```python
from build123d import *

# Parameters (mm, degrees)
SKETCH1_R      = 1
EXTRUDE2_DEPTH = 5
FILLET2_R      = 3.5
FILLET3_R      = 1.5
EXTRUDE4_DEPTH = 5
FILLET4_R      = 0.2
EXTRUDE5_DEPTH = 5
FILLET5_R      = 0.2


with BuildPart() as part:
    # Sketch1 → Extrude2 (new body)
    with BuildSketch(Plane.XY):
        with BuildLine():
            Line((-30.522603834, 36.180351438), (-30.522603834, 45.180351438))
            Line((-30.522603834, 45.180351438), (-25.522603834, 45.180351438))
            Line((-25.522603834, 45.180351438), (-7.022603834, 0.180351438))
            Line((-7.022603834, 0.180351438), (-30.522603834, 0.180351438))
            Line((-30.522603834, 0.180351438), (-30.522603834, 10.180351438))
            ThreePointArc((-30.522603834, 10.180351438), (-27.540232283, 23.180351438), (-30.522603834, 36.180351438))
        make_face()
        with Locations((-23.522603834, 3.680351438)):
            Circle(SKETCH1_R, mode=Mode.SUBTRACT)
        with Locations((-11.522603834, 3.680351438)):
            Circle(SKETCH1_R, mode=Mode.SUBTRACT)
    extrude(amount=EXTRUDE2_DEPTH)

    # Fillet2
    fillet2_edges = [part.edges().sort_by_distance(p)[0] for p in [
        (-7.022603834, 0.180351438, 2.5),
    ]]
    fillet(fillet2_edges, radius=FILLET2_R)

    # Fillet3
    fillet3_edges = [part.edges().sort_by_distance(p)[0] for p in [
        (-25.522603834, 45.180351438, 2.5),
    ]]
    fillet(fillet3_edges, radius=FILLET3_R)

    # Sketch3 → Extrude4 (cut)
    with BuildSketch(Plane.XY.offset(5)):
        Polygon((-29.822603834, 43.080351438), (-30.522603834, 43.780351438), (-30.522603834, 42.380351438), align=None)
        Polygon((-29.822603834, 44.480351438), (-30.522603834, 45.180351438), (-30.522603834, 43.780351438), align=None)
        Polygon((-29.822603834, 41.680351438), (-30.522603834, 42.380351438), (-30.522603834, 40.980351438), align=None)
        Polygon((-29.822603834, 40.280351438), (-30.522603834, 40.980351438), (-30.522603834, 39.580351438), align=None)
        Polygon((-29.822603834, 38.880351438), (-30.522603834, 39.580351438), (-30.522603834, 38.180351438), align=None)
        Polygon((-29.822603834, 37.480351438), (-30.522603834, 38.180351438), (-30.522603834, 36.780351438), align=None)
    extrude(amount=-EXTRUDE4_DEPTH, mode=Mode.SUBTRACT)

    # Fillet4
    fillet4_edges = [part.edges().sort_by_distance(p)[0] for p in [
        (-30.522603834, 45.180351438, 2.5),
        (-29.822603834, 43.080351438, 2.5),
        (-30.522603834, 42.380351438, 2.5),
        (-30.522603834, 43.780351438, 2.5),
        (-29.822603834, 44.480351438, 2.5),
        (-29.822603834, 41.680351438, 2.5),
        (-30.522603834, 40.980351438, 2.5),
        (-29.822603834, 40.280351438, 2.5),
        (-30.522603834, 39.580351438, 2.5),
        (-29.822603834, 38.880351438, 2.5),
        (-30.522603834, 38.180351438, 2.5),
        (-29.822603834, 37.480351438, 2.5),
        (-30.522603834, 36.780351438, 2.5),
    ]]
    fillet(fillet4_edges, radius=FILLET4_R)

    # Sketch4 → Extrude5 (cut)
    with BuildSketch(Plane.XY.offset(5)):
        Polygon((-29.822603834, 1.080351438), (-30.522603834, 1.780351438), (-30.522603834, 0.380351438), align=None)
        Polygon((-29.822603834, 2.480351438), (-30.522603834, 3.180351438), (-30.522603834, 1.780351438), align=None)
        Polygon((-29.822603834, 3.880351438), (-30.522603834, 4.580351438), (-30.522603834, 3.180351438), align=None)
        Polygon((-29.822603834, 5.280351438), (-30.522603834, 5.980351438), (-30.522603834, 4.580351438), align=None)
        Polygon((-29.822603834, 6.680351438), (-30.522603834, 7.380351438), (-30.522603834, 5.980351438), align=None)
        Polygon((-29.822603834, 8.080351438), (-30.522603834, 8.780351438), (-30.522603834, 7.380351438), align=None)
        Polygon((-29.822603834, 9.480351438), (-30.522603834, 10.180351438), (-30.522603834, 8.780351438), align=None)
    extrude(amount=-EXTRUDE5_DEPTH, mode=Mode.SUBTRACT)

    # Fillet5
    fillet5_edges = [part.edges().sort_by_distance(p)[0] for p in [
        (-30.522603834, 10.180351438, 2.5),
        (-29.822603834, 2.480351438, 2.5),
        (-30.522603834, 1.780351438, 2.5),
        (-29.822603834, 3.880351438, 2.5),
        (-30.522603834, 3.180351438, 2.5),
        (-29.822603834, 5.280351438, 2.5),
        (-30.522603834, 4.580351438, 2.5),
        (-29.822603834, 6.680351438, 2.5),
        (-30.522603834, 5.980351438, 2.5),
        (-29.822603834, 8.080351438, 2.5),
        (-30.522603834, 7.380351438, 2.5),
        (-29.822603834, 9.480351438, 2.5),
        (-30.522603834, 8.780351438, 2.5),
        (-29.822603834, 1.080351438, 2.5),
        (-30.522603834, 0.380351438, 2.5),
    ]]
    fillet(fillet5_edges, radius=FILLET5_R)


solid = part.part
```
Design review of the part built by this model. Coordinates are the model's own, in mm. Coordinates: 2 decimals unless noted, no trailing zeros. Order: outer loops, then holes, each group sorted by start corner. A loop starts at its lowest first (then second) coordinate and runs counter-clockwise, first axis right, second up. Notation, with made-up numbers: (34, -38) -> (55, -38) arc R13 ccw to (55, -16) -> close; hole circle Ø8 at (47, 1.25). An arc over 180 degrees is marked (long way). One line per item, written item: value. Start each with the question number.
Q1. Take a section at D-D, the plane z = 1.15. Give the number of separate pieces and of enclosed holes in the cut face, then the cut area to 3 significant figures.
Q2. Insertion check: pin 1 Ø1 at (x, z) = (-21, 4.5) entering from +Y; pin 2 Ø1 at (y, z) = (10.5, 1) entering from +X. Each pin has a flat end and moves straight along its axis. Give the tip position at first contact, or say it passes through.
Q3. For probe 1 along X at (y, z) = (4.5, 2.8); probe 2 along X at (y, z) = (3.5, 0.8); probe 3 along Y at (x, z) = (-24.25, 4.65), list the stretches that pass through material, from the lowest coordinate up.
Q4. Take a section at C-C, the plane y = 23. State the section outline as (x, z) points, then the cut area to 3 significant figures.
Q5. Take a section at A-A, the plane x = -11.5. State the section outline as (y, z) points, then the cut area to 3 significant figures.
Q6. Mouldability with a two-part tool opening along X and no side actions: class faces 1 (the flat face through (-22, 18, 5)), 2 (the cylindrical face through (-25.68, 44.92, 2.54)), 3 (the cylindrical face through (-27.54, 23.06, 2.46)), 4 (the cylindrical face through (-10.599, 3.297, 2.465)) as pulls with the +X half, pulls with the -X half, needs draft (parallel to the pull), parting line crosses it, or undercut.
Q7. Take a section at B-B, the plane x = -28.25. State the section outline as (y, z) points.
Values follow:
1. separate pieces: 1
1. enclosed holes: 2
1. area: 570 mm2
2. pin 1: stops at y = 35.4
2. pin 2: stops at x = -11.06
3. probe 1: x = -30.42 to -24.1, -22.95 to -12.1, -10.95 to -8.84
3. probe 2: x = -30.2 to -24.51, -22.54 to -12.51, -10.54 to -8.75
3. probe 3: y = 0.18 to 2.99, 4.37 to 42.08
4. outline: (-27.54, 0) -> (-16.4, 0) -> (-16.4, 5) -> (-27.54, 5) -> close
4. area: 55.7 mm2
5. outline: (0.26, 0) -> (2.68, 0) -> (2.68, 5) -> (0.26, 5) -> close; (4.68, 0) -> (11.07, 0) -> (11.07, 5) -> (4.68, 5) -> close
5. area: 44.1 mm2
6. face 1: needs draft
6. face 2: pulls with the +X half
6. face 3: pulls with the -X half
6. face 4: undercut
7. outline: (0.18, 0) -> (16.71, 0) -> (16.71, 5) -> (0.18, 5) -> close; (29.65, 0) -> (45.18, 0) -> (45.18, 5) -> (29.65, 5) -> close
